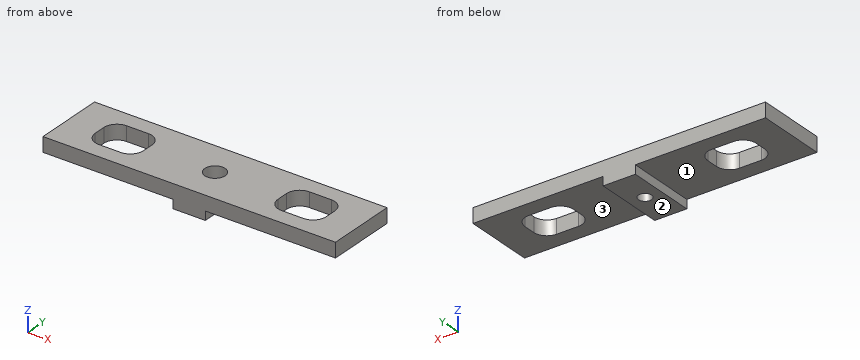
from build123d import *

# Parameters (mm, degrees)
F1_DEPTH = 48
F3_DEPTH = 10
F2_R     = 7
F2_R_2   = 4.5
F4_DEPTH = 10
F5_DEPTH = 25


with BuildPart() as f1:
    # F0 (on Front) → F1 (new body)
    with BuildSketch(Plane.XZ):
        Polygon((-100, 0), (-11, 0), (-11, -6), (11, -6), (11, 0), (100, 0), (100, 10), (-100, 10), align=None)
    extrude(amount=F1_DEPTH)

    # F2 (on face) → F3 (cut)
    with BuildSketch(Plane.XY.offset(10)):
        with BuildLine():
            Line((-78.960404, -19.989976), (-78.960404, -27.985966))
            ThreePointArc((-78.960404, -27.985966), (-76.325687, -34.346737), (-69.964915, -36.981455))
            Line((-69.964915, -36.981455), (-54.972433, -36.981455))
            ThreePointArc((-54.972433, -36.981455), (-48.611662, -34.346737), (-45.976944, -27.985966))
            Line((-45.976944, -27.985966), (-45.976944, -19.989976))
            ThreePointArc((-45.976944, -19.989976), (-48.611662, -13.629204), (-54.972433, -10.994487))
            Line((-54.972433, -10.994487), (-69.964915, -10.994487))
            ThreePointArc((-69.964915, -10.994487), (-76.325687, -13.629204), (-78.960404, -19.989976))
        make_face()
        with BuildLine():
            ThreePointArc((45.976944, -27.985966), (48.611662, -34.346737), (54.972433, -36.981455))
            Line((54.972433, -36.981455), (69.964915, -36.981455))
            ThreePointArc((69.964915, -36.981455), (76.325687, -34.346737), (78.960404, -27.985966))
            Line((78.960404, -27.985966), (78.960404, -19.989976))
            ThreePointArc((78.960404, -19.989976), (76.325687, -13.629204), (69.964915, -10.994487))
            Line((69.964915, -10.994487), (54.972433, -10.994487))
            ThreePointArc((54.972433, -10.994487), (48.611662, -13.629204), (45.976944, -19.989976))
            Line((45.976944, -19.989976), (45.976944, -27.985966))
        make_face()
    extrude(amount=-F3_DEPTH, mode=Mode.SUBTRACT)

    # F2 (on face) → F4 (cut)
    with BuildSketch(Plane.XY.offset(10)):
        with Locations((0, -24)):
            Circle(F2_R)
        with Locations((0, -24)):
            Circle(F2_R_2, mode=Mode.SUBTRACT)
    extrude(amount=-F4_DEPTH, mode=Mode.SUBTRACT)

    # F2 (on face) → F5 (cut)
    with BuildSketch(Plane.XY.offset(10)):
        with Locations((0, -24)):
            Circle(F2_R_2)
    extrude(amount=-F5_DEPTH, mode=Mode.SUBTRACT)


solid = f1.part
For this review, take the finished solid that the model builds, in its own axes (mm). Face numbers are marked on the shaded views. A direction names the side the tool comes from. Round coordinates to 2 decimals unless told otherwise and drop trailing zeros. Order: outer loops, then holes, each group sorted by start corner. A loop starts at its lowest first (then second) coordinate and runs counter-clockwise, first axis right, second up. Notation, with made-up numbers: (18.25, -16) -> (47.25, -16) arc R21 ccw to (47.25, 22) -> close; hole circle Ø2 at (-13.75, 9.5). An arc over 180 degrees is marked (long way). Put each result on its own line as item: value.
Q1. Add section B-B on y = -24. Write out the cut boundary in (x, z).
Check result:
outline: (-100, 0) -> (-78.96, 0) -> (-78.96, 10) -> (-100, 10) -> close; (-45.98, 0) -> (-11, 0) -> (-11, -6) -> (-4.5, -6) -> (-4.5, 0) -> (-7, 0) -> (-7, 10) -> (-45.98, 10) -> close; (4.5, -6) -> (11, -6) -> (11, 0) -> (45.98, 0) -> (45.98, 10) -> (7, 10) -> (7, 0) -> (4.5, 0) -> close; (78.96, 0) -> (100, 0) -> (100, 10) -> (78.96, 10) -> close
Q2. For probe 1 along Y at (x, z) = (0, 7.25); probe 2 along Y at (x, z) = (-0.5, -4); probe 3 along Z at (x, y) = (-34, -45), list the stretches that pass through material, from the lowest coordinate up. Write a range as [from, to].
Check result:
probe 1: [-48, -31], [-17, 0]
probe 2: [-48, -28.47], [-19.53, 0]
probe 3: [0, 10]
Q3. Insertion check: pin 1 Ø8 at (x, y) = (0, -24) entering from -Z; pin 2 Ø2 at (x, y) = (-33.5, -15.5) entering from -Z; pin 3 Ø1.8 at (y, z) = (-31, -3.5) entering from -X; pin 4 Ø4 at (x, y) = (-0.5, -27) entering from +Z. Each pin has a flat end and moves straight along its axis. Give the tip position at first contact, or say it passes through.
Check result:
pin 1: through
pin 2: z = 0
pin 3: x = -11
pin 4: z = 0
Q4. Add section A-A on z = 6.25. Write out the cut boundary in (x, y).
Check result:
outline: (-100, -48) -> (100, -48) -> (100, 0) -> (-100, 0) -> close; hole (-78.96, -27.99) arc R9 ccw to (-69.96, -36.98) -> (-54.97, -36.98) arc R9 ccw to (-45.98, -27.99) -> (-45.98, -19.99) arc R9 ccw to (-54.97, -10.99) -> (-69.96, -10.99) arc R9 ccw to (-78.96, -19.99) -> close; hole circle Ø14 at (0, -24); hole (45.98, -27.99) arc R9 ccw to (54.97, -36.98) -> (69.96, -36.98) arc R9 ccw to (78.96, -27.99) -> (78.96, -19.99) arc R9 ccw to (69.96, -10.99) -> (54.97, -10.99) arc R9 ccw to (45.98, -19.99) -> close
Q5. Add section D-D on z = -2.5. Write out the cut boundary in (x, y), plus the area to 3 significant figures.
Check result:
outline: (-11, -48) -> (11, -48) -> (11, 0) -> (-11, 0) -> close; hole circle Ø9 at (0, -24)
area: 992 mm2
Q6. Add section C-C on x = 63. Write out the cut boundary in (y, z), plus the area to 3 significant figures.
Check result:
outline: (-48, 0) -> (-36.98, 0) -> (-36.98, 10) -> (-48, 10) -> close; (-10.99, 0) -> (0, 0) -> (0, 10) -> (-10.99, 10) -> close
area: 220 mm2
Q7. Machinability: for the marked faces 1, 2 and 3, which of the approach directions +Z, -Z, +X, -X, +Y, -Y give a long, thin tool a straight path to every point of the face, cutting with its end or side? Answer none if there is none.
Check result:
face 1: -Z, -X, +Y, -Y
face 2: -Z, +X, -X, +Y, -Y
face 3: -Z, +X, +Y, -Y
